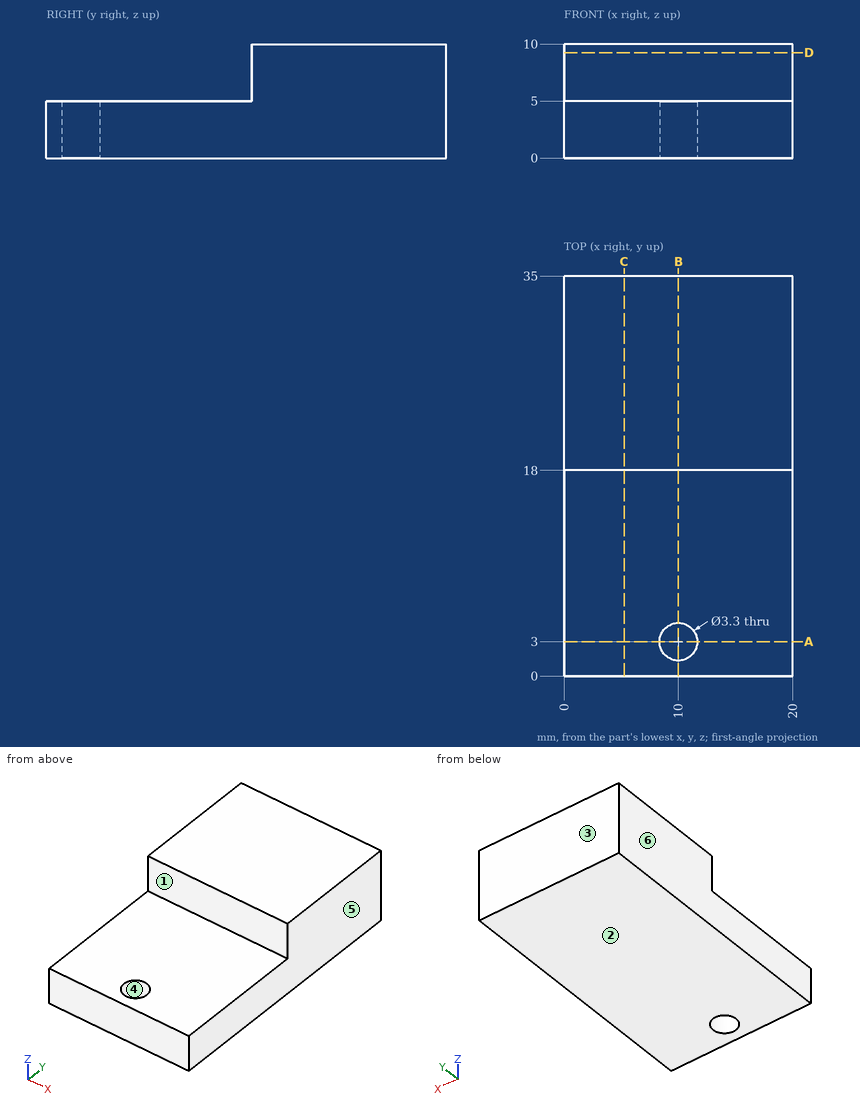
Design review of the part shown in the three views and the two pictorial views. Dimensions are in mm from the part's minimum x, y and z. A direction names the side the tool comes from. Round coordinates to 2 decimals unless told otherwise and drop trailing zeros. Loops run counter-clockwise (first coordinate to the right, second up) from the corner with the lowest first, then second, coordinate; pieces in that order, holes last. Notation, with made-up numbers: (-23.75, 7.25) -> (-7.75, 7.25) arc R21 cw to (-7.75, 46.25) -> close; hole circle Ø5 at (-8, 49.5). An arc over 180 degrees is marked (long way). Use one line per item in the form item = value. Start each with the question number.
Q1. Wall thickness on line 1 along X through (y, z) = (3, 3.2); line 2 along Y through (x, z) = (10, 3.25); line 3 along Y through (x, z) = (1, 8): over which ranges is each line inside the solid? List them lowest first. Write a range as [from, to].
Q2. We need section A-A on y = 3. Give the boundary of the cut face in (x, z), then the cut area to 3 significant figures.
Q3. Machinability: for the marked faces 1 and 2, which of the approach directions +Z, -Z, +X, -X, +Y, -Y give a long, thin tool a straight path to every point of the face, cutting with its end or side? Answer none if there is none.
Q4. Draft analysis for pull direction X (two halves, no side actions). For the marked faces 3, 4, 5 and 6, state which applies: +X half, -X half, draft (parallel to the pull), parting line (faces both ways), or undercut.
Q5. For pin 1 Ø10 at (x, y) = (7.5, 29.5) entering from -Z, flat-tipped, find the tip position at first contact; note if it passes through.
Q6. We need section C-C on x = 5.25. Give the boundary of the cut face in (y, z).
Q7. We need section B-B on x = 10. Give the boundary of the cut face in (y, z).
Q8. We need section D-D on z = 9.25. Give the boundary of the cut face in (x, y).
Calculated:
q1.line_1 = [0, 8.35], [11.65, 20]
q1.line_2 = [0, 1.35], [4.65, 35]
q1.line_3 = [18, 35]
q2.outline = (0, 0) -> (8.35, 0) -> (8.35, 5) -> (0, 5) -> close; (11.65, 0) -> (20, 0) -> (20, 5) -> (11.65, 5) -> close
q2.area = 83.5 mm²
q3.face_1 = +Z, +X, -X, -Y
q3.face_2 = -Z, +X, -X, +Y, -Y
q4.face_3 = draft
q4.face_4 = undercut
q4.face_5 = +X half
q4.face_6 = -X half
q5.pin_1 = 0
q6.outline = (0, 0) -> (35, 0) -> (35, 10) -> (18, 10) -> (18, 5) -> (0, 5) -> close
q7.outline = (0, 0) -> (1.35, 0) -> (1.35, 5) -> (0, 5) -> close; (4.65, 0) -> (35, 0) -> (35, 10) -> (18, 10) -> (18, 5) -> (4.65, 5) -> close
q8.outline = (0, 18) -> (20, 18) -> (20, 35) -> (0, 35) -> close
